Check sheet for the modelled part. Datum: model origin and axes. Units: mm. Face numbers are marked on the shaded views. A direction names the side the tool comes from. Give positions to 0.01 mm unless a question says otherwise; leave off trailing zeros. Order: outer loops, then holes, each group sorted by start corner. A loop starts at its lowest first (then second) coordinate and runs counter-clockwise, first axis right, second up. Notation, with made-up numbers: (70.5, 48.25) -> (86.5, 48.25) arc R35 ccw to (86.5, 86.25) -> close; hole circle Ø6 at (-22, 34). An arc over 180 degrees is marked (long way). One line per question, with ' | ' between items.
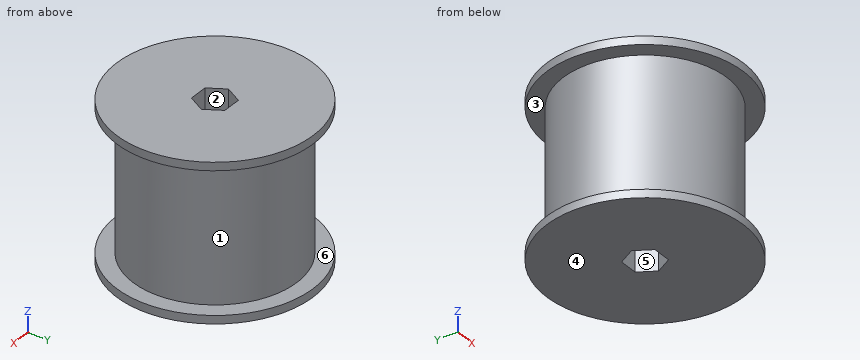
Autodesk Inventor part; units mm, degrees
ref_plane "YZ Plane" through (0, 0, 0) normal (1, 0, 0) x (0, 1, 0)
ref_plane "XZ Plane" through (0, 0, 0) normal (0, 1, 0) x (-1, 0, 0)
ref_plane "XY Plane" through (0, 0, 0) normal (0, 0, 1) x (1, 0, 0)
sketch "Sketch1" plane through (0, 0, 0) normal (0, 1, 0) x (-1, 0, 0)
  line L0 (31.75, -26.9875) -> (0, -26.9875)
  line L1 (0, -26.9875) -> (0, 26.9875)
  line L2 (0, 26.9875) -> (31.75, 26.9875)
  line L3 (31.75, 26.9875) -> (31.75, -26.9875)
  line L4 (0, -26.9875) -> (38.1, -26.9875)
  line L5 (38.1, -26.9875) -> (38.1, -30.1625)
  line L6 (38.1, -30.1625) -> (0, -30.1625)
  line L7 (0, -30.1625) -> (0, -26.9875)
  line L8 (0, 26.9875) -> (38.1, 26.9875)
  line L9 (38.1, 26.9875) -> (38.1, 30.1625)
  line L10 (38.1, 30.1625) -> (0, 30.1625)
  line L11 (0, 30.1625) -> (0, 26.9875)
  line L12 (0, 0) -> (51.6774, 0) construction
  point P0 (31.75, -26.9875)
  point P1 (31.75, 26.9875)
  dimension "d0" = 53.975
  dimension "d1" = 6.35
  dimension "d2" = 60.325
  dimension "d4" = 31.75
revolve "Revolution1" add sketch "Sketch1" angle 360 about axis through (0, 0, -26.9875) along (0, 0, 1)
sketch "Sketch2" plane through (0, 0, 30.1625) normal (0, 0, 1) x (1, 0, 0)
  line L0 (7.479, 0) -> (3.7395, -6.477)
  line L1 (3.7395, -6.477) -> (-3.7395, -6.477)
  line L2 (-3.7395, -6.477) -> (-7.479, 0)
  line L3 (-7.479, 0) -> (-3.7395, 6.477)
  line L4 (-3.7395, 6.477) -> (3.7395, 6.477)
  line L5 (3.7395, 6.477) -> (7.479, 0)
  point P0 (0, 0)
  point P1 (0, 0)
  point P2 (0, 6.477)
  dimension "d6" = 12.954
extrude "Extrusion1" cut sketch "Sketch2" against normal through all
equation "\"d4\" = d9"
equation "\"d9\" = 31.75"
properties part number "Polybelt Wheels" material "ABS Plastic"
Q1. Access from +Z, -Z, +X, -X, +Y, -Y to the whole of each face (thin tool, end or side, straight path). Record for the marked faces 4, 5 and 6.
Result sheet:
face 4: -Z, +X, -X, +Y, -Y | face 5: +Z, -Z | face 6: none
Q2. Mould release check, pull along Y, two halves, no side actions. Record for the marked faces 1, 2 and 3: pulls with the +Y half, pulls with the -Y half, needs draft (parallel to the pull), parting line crosses it, or undercut.
Result sheet:
face 1: parting line crosses it | face 2: undercut | face 3: needs draft
Q3. Thickness scan on line 1 (X direction, y = 0, z = 2.5); line 2 (Z direction, x = 32.5, y = 1.5); line 3 (X direction, y = 4, z = 16). Record the ranges inside material, lowest first.
Result sheet:
line 1: x = -31.75 to -7.48, 7.48 to 31.75 | line 2: z = -30.16 to -26.99, 26.99 to 30.16 | line 3: x = -31.5 to -5.17, 5.17 to 31.5
Q4. Section check D-D (y = -30.5). Enter the section's corners in (x, z), and give its area (3 significant figures).
Result sheet:
outline: (-22.83, -30.16) -> (22.83, -30.16) -> (22.83, -26.99) -> (8.82, -26.99) -> (8.82, 26.99) -> (22.83, 26.99) -> (22.83, 30.16) -> (-22.83, 30.16) -> (-22.83, 26.99) -> (-8.82, 26.99) -> (-8.82, -26.99) -> (-22.83, -26.99) -> close | area: 1,240 mm2
Q5. Section check C-C (y = 3.5). Enter the section's corners in (x, z), and give its area (3 significant figures).
Result sheet:
outline: (-37.94, -30.16) -> (-5.46, -30.16) -> (-5.46, 30.16) -> (-37.94, 30.16) -> (-37.94, 26.99) -> (-31.56, 26.99) -> (-31.56, -26.99) -> (-37.94, -26.99) -> close; (5.46, -30.16) -> (37.94, -30.16) -> (37.94, -26.99) -> (31.56, -26.99) -> (31.56, 26.99) -> (37.94, 26.99) -> (37.94, 30.16) -> (5.46, 30.16) -> close | area: 3,230 mm2
Q6. Section check A-A (x = 0). Enter the section's corners in (y, z), and give its area (3 significant figures).
Result sheet:
outline: (-38.1, -30.16) -> (-6.48, -30.16) -> (-6.48, 30.16) -> (-38.1, 30.16) -> (-38.1, 26.99) -> (-31.75, 26.99) -> (-31.75, -26.99) -> (-38.1, -26.99) -> close; (6.48, -30.16) -> (38.1, -30.16) -> (38.1, -26.99) -> (31.75, -26.99) -> (31.75, 26.99) -> (38.1, 26.99) -> (38.1, 30.16) -> (6.48, 30.16) -> close | area: 3,130 mm2
Q7. Section check B-B (z = -14). Enter the section's corners in (x, y), and give its area (3 significant figures).
Result sheet:
outline: circle Ø63.5 at (0, 0); hole (-7.48, 0) -> (-3.74, -6.48) -> (3.74, -6.48) -> (7.48, 0) -> (3.74, 6.48) -> (-3.74, 6.48) -> close | area: 3,020 mm2
Q8. Depth check by flat-ended pin: pin 1 Ø8 at (x, z) = (-0.5, -10.5) entering from -Y; pin 2 Ø4 at (x, z) = (-2.5, -5.5) entering from +Y; pin 3 Ø2 at (x, z) = (22, 11.5) entering from -Y. Enter the tip coordinate at first touch or a pass-through.
Result sheet:
pin 1: stops at y = -31.75 | pin 2: stops at y = 31.75 | pin 3: stops at y = -23.81
